Work out the finished part from the listing and answer in its coordinate system (mm). A direction names the side the tool comes from. Round coordinates to 2 decimals unless told otherwise and drop trailing zeros. Write each loop counter-clockwise with the first axis right and the second up, starting at its lowest first coordinate (ties: lowest second). Pieces come first, ordered by that corner, then holes. Notation, with made-up numbers: (30, 13) -> (40, 13) arc R24 ccw to (40, 31) -> close; hole circle Ø7 at (4, 36.5). An arc over 180 degrees is marked (long way). One line per item, written item: value.
Autodesk Inventor part; units mm, degrees
ref_plane "Work Plane1" through (29, 0, 0) normal (0, -1, 0) x (1, 0, 0)
ref_plane "YZ Plane" through (0, 0, 0) normal (1, 0, 0) x (0, 1, 0)
ref_plane "XZ Plane" through (0, 0, 0) normal (0, 1, 0) x (-1, 0, 0)
sketch "Sketch1" plane through (0, 0, 0) normal (0, 0, 1) x (1, 0, 0)
  line L0 (-1.2192, 0) -> (57.15, 0)
  line L1 (57.15, 0) -> (57.15, 2.413)
  line L2 (57.15, 2.413) -> (35.052, 2.413)
  line L3 (35.052, 2.413) -> (32.406, 2.413)
  line L4 (32.406, 2.413) -> (0, 2.413)
  line L5 (0, 2.413) -> (0, 3.9624)
  line L6 (0, 3.9624) -> (-4.826, 3.9624)
  line L7 (-4.826, 3.9624) -> (-4.826, 2.2877)
  line L8 (-4.826, 2.2877) -> (-2.54, 2.2877)
  line L9 (-2.54, 2.2877) -> (-1.2192, 0)
  line L10 (-17.2212, 0) -> (69.5452, 0)
  line L11 (0, -0.7925) -> (0, 4.7549)
  line L12 (35.052, 2.413) -> (0, 2.413) construction
  dimension "d1" = 22.098
  dimension "d2" = 2.646
  dimension "d3" = 4.826
  dimension "d4" = 2.286
  dimension "d5" = 60
  dimension "d6" = 4.826
  dimension "d7" = 4.826
  dimension "d8" = 4.5754
  dimension "d9" = 7.9248
  dimension "d26" = 57.15
revolve "Body" add sketch "Sketch1" angle 360 about axis through (-1.2192, 0, 0) along (1, 0, 0)
sketch "Sketch2" plane through (-4.826, 0, 0) normal (-1, 0, 0) x (0, 0, 1)
  circle A0 centre (0, 0) radius 2.2877
  line L0 (0, -5.5474) -> (0, 5.5474)
  line L1 (-5.5474, 0) -> (5.5474, 0)
  line L2 (2.2877, 0) -> (1.1438, -1.9812)
  line L3 (1.1438, -1.9812) -> (-1.1438, -1.9812)
  line L4 (-1.1438, -1.9812) -> (-2.2877, 0)
  line L5 (-2.2877, 0) -> (-1.1438, 1.9812)
  line L6 (-1.1438, 1.9812) -> (1.1438, 1.9812)
  line L7 (1.1438, 1.9812) -> (2.2877, 0)
extrude "Slot" add sketch "Sketch2" against normal up to next contours L7 A0 | A0 L2 | L6 L0 A0 | A0 L0 L3 | L0 L6 A0 | A0 L3 L0 | L4 A0 | A0 L5
fillet "Fillet1" radius 0.4572 1 edges at (-4.826, -3.9624, 0)
thread "Thread"
chamfer "Chamfer1" distance 0.6299 distance2 0.6299 1 edges at (57.15, -2.413, 0) measured on face at (57.15, -0.4231, -0.1925)
ref_plane "Work Plane1" through (29, 0, 0) normal (0, -1, 0) x (1, 0, 0)
fillet "Fillet2" radius 0.1524 1 edges at (0, -2.413, 0)
equation "\"d1\" = GEL"
equation "\"d3\" = KOH"
equation "\"d4\" = INTI"
equation "\"d6\" = GD"
equation "\"d7\" = BDM"
equation "\"d8\" = 1.1547 * SW"
equation "\"d9\" = KOD"
equation "\"d26\" = NLG"
equation "\"d30\" = R"
equation "\"d17\" = RR"
equation "\"d13\" = GEL"
equation "\"d15\" = -0.5 * SPD + 0.5 * GD"
equation "\"d16\" = GUL"
equation "\"GD\" = 4.826"
equation "\"NLG\" = 57.15"
equation "\"GEL\" = 22.098"
equation "\"KOD\" = 7.9248"
equation "\"KOH\" = 4.826"
equation "\"INTI\" = 2.286"
equation "\"GAL\" = 2.64592"
equation "\"GUL\" = 0.62992"
equation "\"BDM\" = 4.826"
equation "\"SW\" = 3.9624"
equation "\"RR\" = 0.4572"
equation "\"SPD\" = 3.56616"
equation "\"R\" = 0.1524"
equation "\"PHH\" = 0.127"
equation "\"GD1\" = SPD"
equation "\"THREADDIA\" = 4.826"
equation "\"FAWI\" = 45deg"
equation "\"KOH1\" = 4.3434"
equation "\"NND\" = 4.826"
equation "\"TOA\" = 30deg"
equation "\"E0\" = 1.155 * SW"
properties part number "ANSI B18.3 - No. 10 - 24 UNC - 2 1/4 HS HCS" material "Steel, Mild"
(1) A tool of negligible diameter and unlimited length cuts with its end or side. For faces 1 (the face through (-4, 1.981, 0)), 2 (the face through (57.15, 0, 0)), from which of +Z, -Z, +X, -X, +Y, -Y can it reach the whole face along a straight path? Write none if from no direction.
Reported:
face 1: -X
face 2: +Z, -Z, +X, +Y, -Y
(2) Find section A-A on x = 31.5. Give the vertices of the cut face in (y, z).
Reported:
outline: circle Ø4.83 at (0, 0)
(3) Consider probe 1 along Y at (x, z) = (21, 0.25); probe 2 along Y at (x, z) = (28, 0.75); probe 3 along Z at (x, y) = (27.5, 0). Determine where each line is inside the solid, lowest interval first.
Reported:
probe 1: y = -2.4 to 2.4
probe 2: y = -2.29 to 2.29
probe 3: z = -2.41 to 2.41
(4) For a pull along Y with two mould halves and no side action, classify faces 3 (the face through (-3.61, 1, 1.71)), 4 (the face through (0, 3, 0)), 5 (the face through (27.942, -1.915, 1.468)), 6 (the face through (-3.61, -1, -1.71)) as pulls with the +Y half, pulls with the -Y half, needs draft (parallel to the pull), parting line crosses it, or undercut.
Reported:
face 3: undercut
face 4: needs draft
face 5: parting line crosses it
face 6: undercut
(5) Flat-ended cylindrical pins translate along their axes: pin 1 Ø1 at (x, y) = (44.5, 1.5) entering from +Z; pin 2 Ø4 at (x, y) = (8, 2.5) entering from -Z; pin 3 Ø1 at (y, z) = (3, 2) entering from +X. Find the tip coordinate at first contact, or state that the pin passes through.
Reported:
pin 1: stops at z = 2.2
pin 2: stops at z = -2.36
pin 3: stops at x = 0
